CAD build for the part. Positions are in the model's coordinates, mm. Give positions to 0.01 mm unless a question says otherwise; leave off trailing zeros. Loops run counter-clockwise (first coordinate to the right, second up) from the corner with the lowest first, then second, coordinate; pieces in that order, holes last.
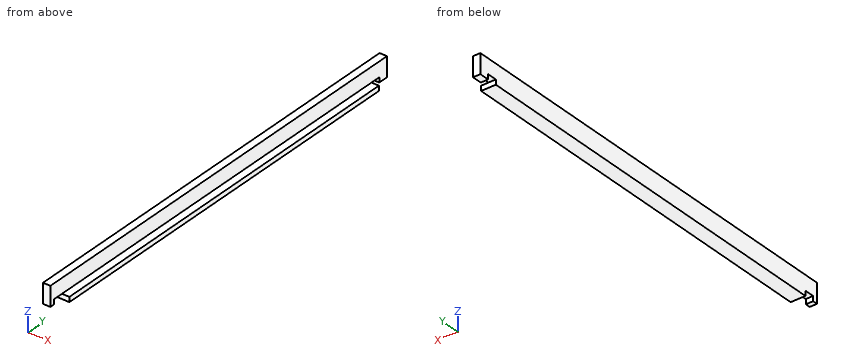
```python
from build123d import *

# Parameters (mm, degrees)
F1_DEPTH = 38.1
F2_W     = 38.1
F2_H     = 25.4
F3_DEPTH = 2133.6
F4_DEPTH = 101.6


with BuildPart() as f1:
    # F0 (on Right) → F1 (new body)
    with BuildSketch(Plane.YZ):
        Polygon((1104.9, 50.8), (-1104.9, 50.8), (-1104.9, -50.8), (-1079.5, -50.8), (-1079.5, -25.4), (-1028.7, -25.4), (-1028.7, -50.8), (1003.3, -50.8), (1003.3, -25.4), (1054.1, -25.4), (1054.1, -50.8), (1104.9, -50.8), align=None)
    extrude(amount=F1_DEPTH)

    # F2 (on face) → F3 (join)
    with BuildSketch(Plane(origin=(0, 1104.9, 0), x_dir=(-1, 0, 0), z_dir=(0, 1, 0))):
        with Locations((-57.15, -38.1)):
            Rectangle(F2_W, F2_H)
    extrude(amount=-F3_DEPTH)

    # F2 (on face) → F4 (cut)
    with BuildSketch(Plane(origin=(0, 1104.9, 0), x_dir=(-1, 0, 0), z_dir=(0, 1, 0))):
        with Locations((-57.15, -38.1)):
            Rectangle(F2_W, F2_H)
    extrude(amount=-F4_DEPTH, mode=Mode.SUBTRACT)


solid = f1.part
```
1. Saw through at B-B, the plane x = 63. List the corners of the cut face in (y, z).
Responses:
outline: (-1028.7, -50.8) - (1003.3, -50.8) - (1003.3, -25.4) - (-1028.7, -25.4) - close
2. Probe line 1 along Y through (x, z) = (37.5, -37); line 2 along X through (y, z) = (772, 6); line 3 along Z through (x, y) = (49, 725). List the from-to ranges inside material, lowest first.
Responses:
line 1: y = -1104.9 to -1079.5, -1028.7 to 1003.3, 1054.1 to 1104.9
line 2: x = 0 to 38.1
line 3: z = -50.8 to -25.4
3. Saw through at A-A, the plane y = 274. List the corners of the cut face in (x, z), and give its area (3 significant figures).
Responses:
outline: (0, -50.8) - (76.2, -50.8) - (76.2, -25.4) - (38.1, -25.4) - (38.1, 50.8) - (0, 50.8) - close
area: 4,840 mm2
4. Drop flat-ended pins along their axis: pin 1 (19 mm diameter, centred on x = 58, y = -303.5, fed in from +Z); pin 2 (11.5 mm diameter, centred on x = 15, y = 1030, fed in from -Z). Give the stop position or say it passes through.
Responses:
pin 1: stops at z = -25.4
pin 2: stops at z = -25.4
5. Saw through at C-C, the plane z = -2. List the corners of the cut face in (x, y), and give its area (3 significant figures).
Responses:
outline: (0, -1104.9) - (38.1, -1104.9) - (38.1, 1104.9) - (0, 1104.9) - close
area: 84,200 mm2
